For this review, take the finished solid that the model builds, in its own axes (mm). Give positions to 0.01 mm unless a question says otherwise; leave off trailing zeros. Loops run counter-clockwise (first coordinate to the right, second up) from the corner with the lowest first, then second, coordinate; pieces in that order, holes last.
```python
from build123d import *

# Parameters (mm, degrees)
SALIENTE_EXTRUIR1_DEPTH = 3
REDONDEO1_R             = 10
CROQUIS2_R              = 1.5
CROQUIS2_R_2            = 2.05
CROQUIS2_W              = 42
CROQUIS2_H              = 20
CORTAR_EXTRUIR1_DEPTH   = 135.610141171
CROQUIS3_W              = 4
CROQUIS3_H              = 14.636342218
CORTAR_EXTRUIR2_DEPTH   = 135.610141171
CROQUIS4_W              = 44
CROQUIS4_H              = 22
CORTAR_EXTRUIR3_DEPTH   = 131.820067673
CORTAR_EXTRUIR4_DEPTH   = 131.820067673
REDONDEO2_R             = 20
CORTAR_EXTRUIR5_DEPTH   = 10
REDONDEO3_R             = 10
CROQUIS7_W              = 14.636342218
CROQUIS7_H              = 3
SALIENTE_EXTRUIR2_DEPTH = 2
CROQUIS8_W              = 14.636342218
CROQUIS8_H              = 3
SALIENTE_EXTRUIR3_DEPTH = 2


with BuildPart() as part:
    # Croquis1 → Saliente-Extruir1 (new body)
    with BuildSketch(Plane(origin=(0, 0, 0), x_dir=(1, 0, 0), z_dir=(0, 1, 0))):
        Polygon((-88.1, 42.318171109), (88.1, 42.318171109), (108.1, 22.318171109), (127.75, 22.318171109), (127.75, 7.681828891), (105.75, 7.681828891), (77.75, -42.318171109), (-77.75, -42.318171109), (-105.75, 7.681828891), (-127.75, 7.681828891), (-127.75, 22.318171109), (-108.1, 22.318171109), align=None)
    extrude(amount=SALIENTE_EXTRUIR1_DEPTH)

    # Redondeo1
    redondeo1_edges = [part.edges().sort_by_distance(p)[0] for p in [
        (-88.1, 1.5, -42.318171109),
        (88.1, 1.5, -42.318171109),
        (108.1, 1.5, -22.318171109),
        (105.75, 1.5, -7.681828891),
        (77.75, 1.5, 42.318171109),
        (-77.75, 1.5, 42.318171109),
        (-105.75, 1.5, -7.681828891),
        (-108.1, 1.5, -22.318171109),
    ]]
    fillet(redondeo1_edges, radius=REDONDEO1_R)

    # Croquis2 → Cortar-Extruir1 (cut, through all)
    with BuildSketch(Plane(origin=(0, 3, 0), x_dir=(1, 0, 0), z_dir=(0, 1, 0))):
        with Locations(Location((70, -27.318171109, 0), (0, 0, 270))):
            Circle(CROQUIS2_R)
        with Locations(Location((-70, -27.318171109, 0), (0, 0, 270))):
            Circle(CROQUIS2_R)
        with Locations(Location((-119.996067812, 15, 0), (0, 0, 270))):
            Circle(CROQUIS2_R)
        with Locations(Location((119.996067812, 15, 0), (0, 0, 270))):
            Circle(CROQUIS2_R)
        with Locations(Location((-11.5, -14.318171109, 0), (0, 0, 270))):
            Circle(CROQUIS2_R)
        with Locations(Location((11.5, -14.318171109, 0), (0, 0, 270))):
            Circle(CROQUIS2_R)
        with Locations(Location((-11.5, -37.318171109, 0), (0, 0, 270))):
            Circle(CROQUIS2_R)
        with Locations(Location((11.5, -37.318171109, 0), (0, 0, 270))):
            Circle(CROQUIS2_R)
        with Locations(Location((-61, 7.318171109, 0), (0, 0, 270))):
            Circle(CROQUIS2_R_2)
        with Locations(Location((-11, 7.318171109, 0), (0, 0, 270))):
            Circle(CROQUIS2_R_2)
        with Locations(Location((-61, 13.318171109, 0), (0, 0, 270))):
            Circle(CROQUIS2_R_2)
        with Locations(Location((-61, 1.318171109, 0), (0, 0, 270))):
            Circle(CROQUIS2_R_2)
        with Locations(Location((-11, 13.318171109, 0), (0, 0, 270))):
            Circle(CROQUIS2_R_2)
        with Locations(Location((-11, 1.318171109, 0), (0, 0, 270))):
            Circle(CROQUIS2_R_2)
        with Locations((-36, 7.318171109)):
            Rectangle(CROQUIS2_W, CROQUIS2_H)
    extrude(amount=-CORTAR_EXTRUIR1_DEPTH, mode=Mode.SUBTRACT)

    # Croquis3 → Cortar-Extruir2 (cut, through all)
    with BuildSketch(Plane(origin=(0, 3, 0), x_dir=(1, 0, 0), z_dir=(0, 1, 0))):
        with Locations((-125.75, 15)):
            Rectangle(CROQUIS3_W, CROQUIS3_H)
        with Locations((125.75, 15)):
            Rectangle(CROQUIS3_W, CROQUIS3_H)
    extrude(amount=-CORTAR_EXTRUIR2_DEPTH, mode=Mode.SUBTRACT)

    # Croquis4 → Cortar-Extruir3 (cut, through all)
    with BuildSketch(Plane(origin=(0, 3, 0), x_dir=(1, 0, 0), z_dir=(0, 1, 0))):
        with Locations((-36, 7.318171109)):
            Rectangle(CROQUIS4_W, CROQUIS4_H)
    extrude(amount=-CORTAR_EXTRUIR3_DEPTH, mode=Mode.SUBTRACT)

    # Croquis5 → Cortar-Extruir4 (cut, through all)
    with BuildSketch(Plane(origin=(0, 3, 0), x_dir=(1, 0, 0), z_dir=(0, 1, 0))):
        Polygon((-63.75, 42.318171109), (-38.75, 32.318171109), (38.75, 32.318171109), (63.75, 42.318171109), align=None)
    extrude(amount=-CORTAR_EXTRUIR4_DEPTH, mode=Mode.SUBTRACT)

    # Redondeo2
    redondeo2_edges = [part.edges().sort_by_distance(p)[0] for p in [
        (-63.75, 1.5, -42.318171109),
        (63.75, 1.5, -42.318171109),
        (38.75, 1.5, -32.318171109),
        (-38.75, 1.5, -32.318171109),
    ]]
    fillet(redondeo2_edges, radius=REDONDEO2_R)

    # Croquis6 → Cortar-Extruir5 (cut)
    with BuildSketch(Plane(origin=(0, 3, 0), x_dir=(1, 0, 0), z_dir=(0, 1, 0))):
        Polygon((-34.898351929, 32.318171109), (-98.1, 32.318171109), (-98.1, 50.604425951), (105.42793471, 50.604425951), (105.42793471, 32.318171109), align=None)
    extrude(amount=-CORTAR_EXTRUIR5_DEPTH, mode=Mode.SUBTRACT)

    # Redondeo3
    redondeo3_edges = [part.edges().sort_by_distance(p)[0] for p in [
        (98.1, 1.5, -32.318171109),
        (-98.1, 1.5, -32.318171109),
    ]]
    fillet(redondeo3_edges, radius=REDONDEO3_R)

    # Croquis7 → Saliente-Extruir2 (add)
    with BuildSketch(Plane.ZY.offset(123.75)):
        with Locations((-15, 1.5)):
            Rectangle(CROQUIS7_W, CROQUIS7_H)
    extrude(amount=SALIENTE_EXTRUIR2_DEPTH)

    # Croquis8 → Saliente-Extruir3 (add)
    with BuildSketch(Plane(origin=(123.75, 0, 0), x_dir=(0, 0, -1), z_dir=(1, 0, 0))):
        with Locations((15, 1.5)):
            Rectangle(CROQUIS8_W, CROQUIS8_H)
    extrude(amount=SALIENTE_EXTRUIR3_DEPTH)


solid = part.part
```
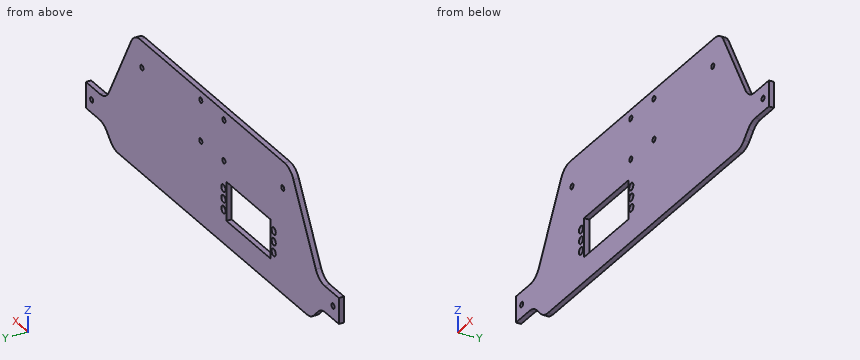
Item 1: For L1, parallel to X at y = 1.55, z = 13; L2, parallel to X at y = 2.6, z = 14; L3, parallel to Z at x = -21.5, y = 0.25, list the stretches that pass through material, from the lowest coordinate up.
Answer:
L1: x = -94.17 to -12.22, -10.78 to 10.78, 12.22 to 94.17
L2: x = -93.61 to -12.97, -10.03 to 10.03, 12.97 to 93.61
L3: z = -32.32 to -18.32, 3.68 to 42.32
Item 2: Take a section at B-B on y = 0.45. State how many separate pieces and enclosed holes the cut face has, and give its area (3 significant figures).
Answer:
separate pieces: 1
enclosed holes: 15
area: 13,800 mm2
Item 3: Clearance check with flat-ended pins moving along their axes: pin 1 Ø0.9 at (x, y) = (119.5, 2) entering from +Z; pin 2 Ø3.5 at (x, z) = (-61, -13.32) entering from -Y; pin 3 Ø0.9 at (x, y) = (121, 1.5) entering from -Z; pin 4 Ø1 at (y, z) = (2.5, 19) entering from +X. State where each tip first meets the part, or that it passes through.
Answer:
pin 1: stops at z = -7.68
pin 2: passes through
pin 3: stops at z = -22.32
pin 4: stops at x = 91.09
Item 4: Take a section at A-A on x = -50.5. Give the boundary of the cut face in (y, z).
Answer:
outline: (0, -32.32) - (3, -32.32) - (3, -18.32) - (0, -18.32) - close; (0, 3.68) - (3, 3.68) - (3, 42.32) - (0, 42.32) - close
